The listing builds one solid part. Answer for the finished solid, in the listing's coordinates (mm). A direction names the side the tool comes from. Give positions to 0.01 mm unless a question says otherwise; leave off trailing zeros. Answer as a JSON object with one key per item and string values. Group by question number.
Q1. Consider line 1 (X direction, y = 162.5, z = 0); line 2 (X direction, y = 15, z = -3); line 3 (X direction, y = 313, z = 6). Determine where each line is inside the solid, lowest interval first.
Q2. The mould has two halves that part along Z. Classify faces 1 (the face through (10, 163, -6)), 2 (the face through (6, 163, -10)), 3 (the face through (6, 163, 10)), 4 (the face through (-5, 168, 0)): released by +Z, released by -Z, zero draft, split by the parting line, or undercut.
Q3. For faces 5 (the face through (-6, 163, 10)), 6 (the face through (0, 168, 5)), determine the directions among +Z, -Z, +X, -X, +Y, -Y from which every point of the face is accessible in a straight line to the end or side of a thin tool.
Q4. Given pin 1 (12 mm diameter, centred on x = -4, z = 0.5, fed in from -Y); pin 2 (1 mm diameter, centred on x = 1.5, y = 89, fed in from -Z), each flat-ended and moving along its own axis, determine where each tip first touches the part or whether it passes through.
from build123d import *

# Parameters (mm, degrees)
SKETCH1_R               = 2.5
BOSS_EXTRUDE1_DEPTH     = 331
ENL_V_MAT_EXTRU_1_DEPTH = 331


with BuildPart() as part:
    # Sketch1 → Boss-Extrude1 (new body)
    with BuildSketch(Plane(origin=(0, 0, 0), x_dir=(1, 0, 0), z_dir=(0, 1, 0))):
        Polygon((2.5, -10), (10, -10), (10, -2.5), (5, -2.5), (5, 2.5), (10, 2.5), (10, 10), (2.5, 10), (2.5, 5), (-2.5, 5), (-2.5, 10), (-10, 10), (-10, 2.5), (-5, 2.5), (-5, -2.5), (-10, -2.5), (-10, -10), (-2.5, -10), (-2.5, -5), (2.5, -5), align=None)
        with Locations(Location((0, 0, 0), (0, 0, 270))):
            Circle(SKETCH1_R, mode=Mode.SUBTRACT)
    extrude(amount=BOSS_EXTRUDE1_DEPTH)

    # Esquisse1 → Enlèv. mat.-Extru.1 (cut)
    with BuildSketch(Plane(origin=(0, 331, 0), x_dir=(1, 0, 0), z_dir=(0, 1, 0))):
        Polygon((-6.585786438, 8.403805922), (-2.5, 8.403805922), (-2.5, 5), (-3.181980515, 5), align=None)
        Polygon((-5, 3.181980515), (-8.403805922, 6.585786438), (-8.403805922, 2.5), (-5, 2.5), align=None)
        Polygon((-3.181980515, -5), (-2.5, -5), (-2.5, -8.403805922), (-6.585786438, -8.403805922), align=None)
        Polygon((-8.403805922, -2.5), (-5, -2.5), (-5, -3.181980515), (-8.403805922, -6.585786438), align=None)
        Polygon((6.585786438, -8.403805922), (2.5, -8.403805922), (2.5, -5), (3.181980515, -5), align=None)
        Polygon((5, -2.5), (5, -3.181980515), (8.403805922, -6.585786438), (8.403805922, -2.5), align=None)
        Polygon((8.403805922, 2.5), (5, 2.5), (5, 3.181980515), (8.403805922, 6.585786438), align=None)
        Polygon((3.181980515, 5), (2.5, 5), (2.5, 8.403805922), (6.585786438, 8.403805922), align=None)
    extrude(amount=-ENL_V_MAT_EXTRU_1_DEPTH, mode=Mode.SUBTRACT)


solid = part.part
Reply:
{
 "1": {"line 1": "x = -5 to -2.5, 2.5 to 5", "line 2": "x = -10 to -8.4, -5 to 5, 8.4 to 10", "line 3": "x = -10 to -8.4, -7.82 to -4.18, 4.18 to 7.82, 8.4 to 10"},
 "2": {"face 1": "zero draft", "face 2": "released by -Z", "face 3": "released by +Z", "face 4": "undercut"},
 "3": {"face 5": "+Z, +X, -X, +Y, -Y", "face 6": "+Y, -Y"},
 "4": {"pin 1": "stops at y = 0", "pin 2": "stops at z = -5"}
}
